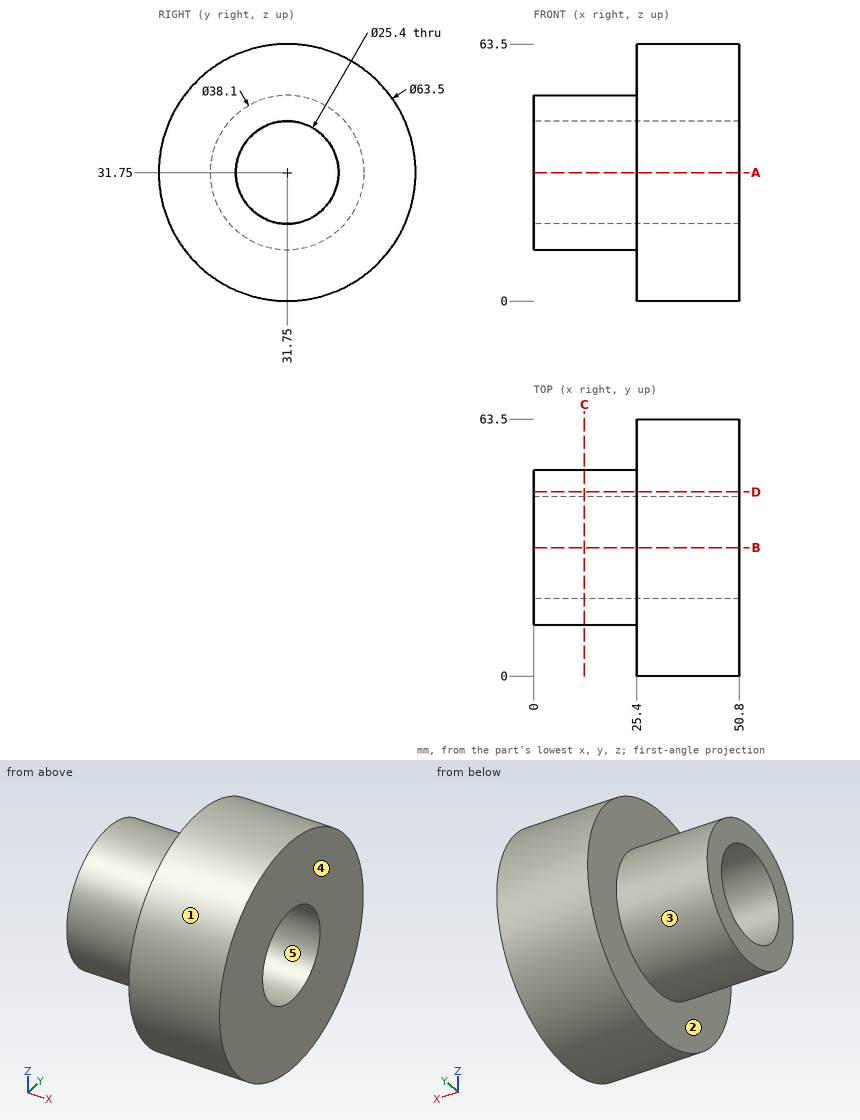
Design review of the part shown in the three views and the two pictorial views. Dimensions are in mm from the part's minimum x, y and z. A direction names the side the tool comes from. Round coordinates to 2 decimals unless told otherwise and drop trailing zeros. Loops run counter-clockwise (first coordinate to the right, second up) from the corner with the lowest first, then second, coordinate; pieces in that order, holes last. Notation, with made-up numbers: (51, -22.75) - (64, -22.75) arc R25 cw to (64, 16.25) - close; hole circle Ø2 at (-10.5, -35). An arc over 180 degrees is marked (long way). Answer as CSV lines item,"result".
(1) Consider section D-D on y = 45.5. Give the boundary of the cut face in (x, z).
Checked values:
outline,"(0, 18.57) - (25.4, 18.57) - (25.4, 3.13) - (50.8, 3.13) - (50.8, 60.37) - (25.4, 60.37) - (25.4, 44.93) - (0, 44.93) - close"
(2) Consider section C-C on x = 12.5. Give the boundary of the cut face in (y, z), then the cut area to 3 significant figures.
Checked values:
outline,"circle Ø38.1 at (31.75, 31.75); hole circle Ø25.4 at (31.75, 31.75)"
area,"633 mm2"
(3) Consider section A-A on z = 31.75. Give the boundary of the cut face in (x, y).
Checked values:
outline,"(0, 12.7) - (25.4, 12.7) - (25.4, 0) - (50.8, 0) - (50.8, 19.05) - (0, 19.05) - close; (0, 44.45) - (50.8, 44.45) - (50.8, 63.5) - (25.4, 63.5) - (25.4, 50.8) - (0, 50.8) - close"
(4) Insertion check: P1, Ø2, axis at y = 54.5, z = 42.5, coming from the -X side; P2, Ø10, axis at x = 33.5, y = 25, coming from the +Z side; P3, Ø10, axis at x = 19.5, z = 22.5, coming from the +Y side; P4, Ø2, axis at x = 13, y = 52, coming from the +Z side. Each pin has a flat end and moves straight along its axis. Give the tip position at first contact, or say it passes through.
Checked values:
P1,"stops at x = 25.4"
P2,"stops at z = 63.45"
P3,"stops at y = 50.32"
P4,"passes through"
(5) Mouldability with a two-part tool opening along Z and no side actions: class the marked faces 3, 4 and 5 as +Z half, -Z half, draft (parallel to the pull), parting line (faces both ways), or undercut.
Checked values:
face 3,"parting line"
face 4,"draft"
face 5,"undercut"
(6) Wall thickness on line 1 (X direction, y = 56.5, z = 14); line 2 (Z direction, x = 20, y = 31); line 3 (Z direction, x = 30, y = 31): over which ranges is each line inside the solid? List them lowest first.
Checked values:
line 1,"x = 25.4 to 50.8"
line 2,"z = 12.71 to 19.07, 44.43 to 50.79"
line 3,"z = 0.01 to 19.07, 44.43 to 63.49"
(7) Tool access review of the marked faces 1 and 2: name each direction out of +Z, -Z, +X, -X, +Y, -Y from which nothing blocks a thin tool from reaching the whole face with its end or side.
Checked values:
face 1,"+X, -X"
face 2,"-X"
